Could you check a few things on this model? Use its own coordinates, in mm. Coordinates: 2 decimals unless noted, no trailing zeros. Order: outer loops, then holes, each group sorted by start corner. A loop starts at its lowest first (then second) coordinate and runs counter-clockwise, first axis right, second up. Notation, with made-up numbers: (-18, 77.25) -> (-12, 77.25) arc R15 cw to (-12, 86.25) -> close; hole circle Ø6 at (-23, 78). An arc over 180 degrees is marked (long way). Put each result on its own line as item: value. Start each with the question number.
Q1. If we section it at A-A (x = 12.7): Please give me the cut outline in (y, z), and give its area (3 significant figures).
Q2. Please list where these lines run through material, in increasing order: line 1 along Y through (x, z) = (12.7, 74.5); line 2 along Y through (x, z) = (15.5, -13); line 3 along X through (y, z) = (216, 1.5).
Q3. If we section it at C-C (y = -233.5): Please give me the cut outline in (x, z).
Q4. If we section it at B-B (z = -11): Count the separate pieces of the cut face and the enclosed holes in it, and give its area (3 significant figures).
Q5. Will these pins go through, and if not, where does the flat tip stop? pin 1 (20.5 mm diameter, centred on y = 359.97, z = 22.39, fed in from -X); pin 2 (15 mm diameter, centred on x = 12.7, y = -325.83, fed in from -Z); pin 3 (1.9 mm diameter, centred on x = -3, y = 239, fed in from +Z); pin 4 (5 mm diameter, centred on x = -3, z = 92.5, fed in from -Y).
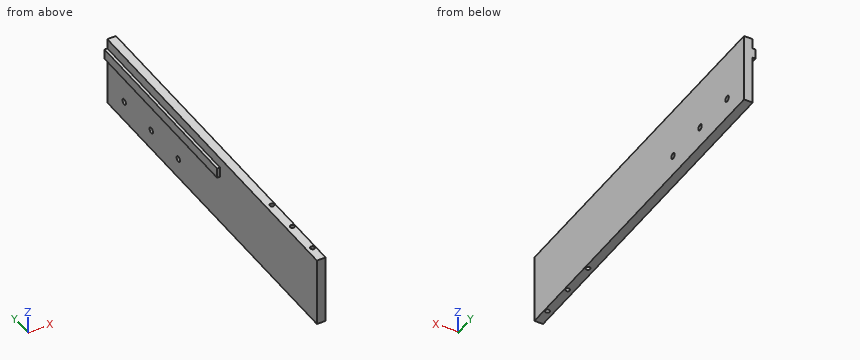
from build123d import *

# Parameters (mm, degrees)
F0_W     = 787.4
F0_H     = 152.4
F1_DEPTH = 19.05
F4_D     = 12.7
F5_D     = 9.525
F6_W     = 423.4667551786
F6_H     = 22.225
F7_DEPTH = 6.35


with BuildPart() as f1:
    # F0 (on Right) → F1 (new body)
    with BuildSketch(Plane.YZ):
        with Locations((29.7667551786, 54.1366326568)):
            Rectangle(F0_W, F0_H)
    extrude(amount=F1_DEPTH)

    # F4 (through all)
    with Locations(Plane.YZ.offset(19.05)):
        with Locations((156.7667551786, 22.3866326568), (258.3667551786, 22.3866326568), (359.9667551786, 22.3866326568)):
            Hole(F4_D / 2)

    # F5 (through all)
    with Locations(Plane.XY.offset(130.3366326568)):
        with Locations((12.7, -173.4332448214), (12.7, -249.6332448214), (12.7, -325.8332448214)):
            Hole(F5_D / 2)

    # F6 (on face) → F7 (join, symmetric)
    with BuildSketch(Plane(origin=(0, 0, 0), x_dir=(0, -1, 0), z_dir=(-1, 0, 0))):
        with Locations((-211.7333775893, 96.9991326568)):
            Rectangle(F6_W, F6_H)
    extrude(amount=F7_DEPTH, both=True)


solid = f1.part
The answers:
1. outline: (-363.93, -22.06) -> (-330.6, -22.06) -> (-330.6, 130.34) -> (-363.93, 130.34) -> close; (-321.07, -22.06) -> (-254.4, -22.06) -> (-254.4, 130.34) -> (-321.07, 130.34) -> close; (-244.87, -22.06) -> (-178.2, -22.06) -> (-178.2, 130.34) -> (-244.87, 130.34) -> close; (-168.67, -22.06) -> (423.47, -22.06) -> (423.47, 130.34) -> (-168.67, 130.34) -> close; hole circle Ø12.7 at (156.77, 22.39); hole circle Ø12.7 at (258.37, 22.39); hole circle Ø12.7 at (359.97, 22.39)
1. area: 115,000 mm^2
2. line 1: -363.93 to -330.6, -321.07 to -254.4, -244.87 to -178.2, -168.67 to 423.47
2. line 2: -363.93 to -329.69, -321.98 to -253.49, -245.78 to -177.29, -169.58 to 423.47
2. line 3: 0 to 19.05
3. outline: (0, -22.06) -> (19.05, -22.06) -> (19.05, 130.34) -> (0, 130.34) -> close
4. separate pieces: 1
4. enclosed holes: 3
4. area: 14,800 mm^2
5. pin 1: x = 0
5. pin 2: z = -22.06
5. pin 3: z = 108.11
5. pin 4: y = 0
